For this review, take the finished solid that the model builds, in its own axes (mm). A direction names the side the tool comes from. Give positions to 0.01 mm unless a question says otherwise; leave off trailing zeros. Order: outer loops, then holes, each group sorted by start corner. A loop starts at its lowest first (then second) coordinate and runs counter-clockwise, first axis right, second up.
from build123d import *

# Parameters (mm, degrees)
F1_DEPTH = 25


with BuildPart() as f1:
    # F0 (on Front) → F1 (new body)
    with BuildSketch(Plane.XZ):
        with BuildLine():
            Line((27.1333980914, 4.2735439138), (-126.4131814241, 56.7106418312))
            Line((-126.4131814241, 56.7106418312), (-126.4131814241, 50.1115843654))
            Line((-126.4131814241, 50.1115843654), (-100.4294008017, -78.9824649692))
            Line((-100.4294008017, -78.9824649692), (109.0906560421, -23.7153619528))
            Line((109.0906560421, -23.7153619528), (31.3300916134, 2.8403473566))
            add(Edge.make_bspline(
                [(31.3300916134, 2.8403473566), (31.6087331931, 2.6379324169), (31.8639740687, 2.4078315454)],
                knots=[0.879679153, 0.879679153, 0.879679153, 1, 1, 1], degree=2))
            add(Edge.make_bspline(
                [(31.8639740687, 2.4078315454), (33.9853094976, 0.4954374993), (33.9853094976, -2.7315460807)],
                knots=[0, 0, 0, 1, 1, 1], degree=2))
            add(Edge.make_bspline(
                [(33.9853094976, -2.7315460807), (33.9853094976, -5.2562544572), (32.5691512359, -7.7229235606)],
                knots=[0, 0, 0, 1, 1, 1], degree=2))
            add(Edge.make_bspline(
                [(32.5691512359, -7.7229235606), (31.1529929742, -10.1895926641), (27.2759695363, -13.9621454105)],
                knots=[0, 0, 0, 1, 1, 1], degree=2))
            Line((27.2759695363, -13.9621454105), (21.4720422341, -19.6383863121))
            Line((21.4720422341, -19.6383863121), (21.4720422341, -19.7834844946))
            Line((21.4720422341, -19.7834844946), (35.1112713943, -19.7834844946))
            Line((35.1112713943, -19.7834844946), (35.1112713943, -22.575173527))
            Line((35.1112713943, -22.575173527), (17.6820777057, -22.575173527))
            Line((17.6820777057, -22.575173527), (17.6820777057, -19.9808180229))
            Line((17.6820777057, -19.9808180229), (24.6642022503, -12.9638699145))
            add(Edge.make_bspline(
                [(24.6642022503, -12.9638699145), (27.8563622665, -9.7310824072), (28.8720495444, -8.3526496729)],
                knots=[0, 0, 0, 1, 1, 1], degree=2))
            add(Edge.make_bspline(
                [(28.8720495444, -8.3526496729), (29.8877368223, -6.9742169386), (30.3955804612, -5.6683332956)],
                knots=[0, 0, 0, 1, 1, 1], degree=2))
            add(Edge.make_bspline(
                [(30.3955804612, -5.6683332956), (30.9034241002, -4.3624496526), (30.9034241002, -2.8592324814)],
                knots=[0, 0, 0, 1, 1, 1], degree=2))
            add(Edge.make_bspline(
                [(30.9034241002, -2.8592324814), (30.9034241002, -0.7349950888), (29.6149522391, 0.5070453539)],
                knots=[0, 0, 0, 1, 1, 1], degree=2))
            add(Edge.make_bspline(
                [(29.6149522391, 0.5070453539), (28.326480378, 1.7490857966), (26.0397330209, 1.7490857966)],
                knots=[0, 0, 0, 1, 1, 1], degree=2))
            add(Edge.make_bspline(
                [(26.0397330209, 1.7490857966), (24.3914176671, 1.7490857966), (22.911416205, 1.2035166302)],
                knots=[0, 0, 0, 1, 1, 1], degree=2))
            add(Edge.make_bspline(
                [(22.911416205, 1.2035166302), (21.4314147429, 0.6579474638), (19.6205894247, -0.7756225799)],
                knots=[0, 0, 0, 1, 1, 1], degree=2))
            Line((19.6205894247, -0.7756225799), (18.0245094165, 1.2731637578))
            add(Edge.make_bspline(
                [(18.0245094165, 1.2731637578), (21.6867875442, 4.3202255915), (26.0049094571, 4.3202255915)],
                knots=[0, 0, 0, 1, 1, 1], degree=2))
            add(Edge.make_bspline(
                [(26.0049094571, 4.3202255915), (26.5888819187, 4.3202255915), (27.1333980914, 4.2735439138)],
                knots=[0, 0, 0, 0.156237232, 0.156237232, 0.156237232], degree=2))
        make_face()
        Polygon((-78.7617822753, 1.2035166302), (-78.7617822753, -22.575173527), (-81.8436676727, -22.575173527), (-81.8436676727, 1.2035166302), (-90.241950479, 1.2035166302), (-90.241950479, 3.9429703168), (-70.3634994689, 3.9429703168), (-70.3634994689, 1.2035166302), align=None, mode=Mode.SUBTRACT)
        Polygon((-51.5877946463, -19.8183080584), (-51.5877946463, -22.575173527), (-66.370397485, -22.575173527), (-66.370397485, 3.9429703168), (-51.5877946463, 3.9429703168), (-51.5877946463, 1.2035166302), (-63.2885120875, 1.2035166302), (-63.2885120875, -7.3398643587), (-52.2958737771, -7.3398643587), (-52.2958737771, -10.0619062634), (-63.2885120875, -10.0619062634), (-63.2885120875, -19.8183080584), align=None, mode=Mode.SUBTRACT)
        with BuildLine():
            add(Edge.make_bspline(
                [(-28.3372618736, 0.1530057885), (-31.3495001434, 1.5633601229), (-34.3617384133, 1.5633601229)],
                knots=[0, 0, 0, 1, 1, 1], degree=2))
            add(Edge.make_bspline(
                [(-34.3617384133, 1.5633601229), (-38.7320956719, 1.5633601229), (-41.2626079756, -1.3473094191)],
                knots=[0, 0, 0, 1, 1, 1], degree=2))
            add(Edge.make_bspline(
                [(-41.2626079756, -1.3473094191), (-43.7931202794, -4.2579789612), (-43.7931202794, -9.3190035687)],
                knots=[0, 0, 0, 1, 1, 1], degree=2))
            add(Edge.make_bspline(
                [(-43.7931202794, -9.3190035687), (-43.7931202794, -14.5193224315), (-41.3525688488, -17.360344846)],
                knots=[0, 0, 0, 1, 1, 1], degree=2))
            add(Edge.make_bspline(
                [(-41.3525688488, -17.360344846), (-38.9120174182, -20.2013672604), (-34.3965619771, -20.2013672604)],
                knots=[0, 0, 0, 1, 1, 1], degree=2))
            add(Edge.make_bspline(
                [(-34.3965619771, -20.2013672604), (-31.6222847266, -20.2013672604), (-28.0644772904, -19.2030917644)],
                knots=[0, 0, 0, 1, 1, 1], degree=2))
            Line((-28.0644772904, -19.2030917644), (-28.0644772904, -21.9019179599))
            add(Edge.make_bspline(
                [(-28.0644772904, -21.9019179599), (-30.8213427589, -22.940820947), (-34.8666800886, -22.940820947)],
                knots=[0, 0, 0, 1, 1, 1], degree=2))
            add(Edge.make_bspline(
                [(-34.8666800886, -22.940820947), (-40.7228427365, -22.940820947), (-43.9062968618, -19.3830135108)],
                knots=[0, 0, 0, 1, 1, 1], degree=2))
            add(Edge.make_bspline(
                [(-43.9062968618, -19.3830135108), (-47.089750987, -15.8252060745), (-47.089750987, -9.2783760776)],
                knots=[0, 0, 0, 1, 1, 1], degree=2))
            add(Edge.make_bspline(
                [(-47.089750987, -9.2783760776), (-47.089750987, -5.1808034023), (-45.5575141793, -2.0989180048)],
                knots=[0, 0, 0, 1, 1, 1], degree=2))
            add(Edge.make_bspline(
                [(-45.5575141793, -2.0989180048), (-44.0252773715, 0.9829673927), (-41.1320196113, 2.6515964921)],
                knots=[0, 0, 0, 1, 1, 1], degree=2))
            add(Edge.make_bspline(
                [(-41.1320196113, 2.6515964921), (-38.2387618512, 4.3202255915), (-34.3211109222, 4.3202255915)],
                knots=[0, 0, 0, 1, 1, 1], degree=2))
            add(Edge.make_bspline(
                [(-34.3211109222, 4.3202255915), (-30.1538911192, 4.3202255915), (-27.0313782306, 2.7995966383)],
                knots=[0, 0, 0, 1, 1, 1], degree=2))
            Line((-27.0313782306, 2.7995966383), (-28.3372618736, 0.1530057885))
        make_face(mode=Mode.SUBTRACT)
        Polygon((-14.1176399831, 1.2035166302), (-14.1176399831, -22.575173527), (-17.1995253806, -22.575173527), (-17.1995253806, 1.2035166302), (-25.5978081869, 1.2035166302), (-25.5978081869, 3.9429703168), (-5.7193571768, 3.9429703168), (-5.7193571768, 1.2035166302), align=None, mode=Mode.SUBTRACT)
        with BuildLine():
            add(Edge.make_bspline(
                [(10.734776725, 2.552929728), (12.8764258995, 0.7856338644), (12.8764258995, -2.2962515331)],
                knots=[0, 0, 0, 1, 1, 1], degree=2))
            add(Edge.make_bspline(
                [(12.8764258995, -2.2962515331), (12.8764258995, -4.8383716914), (11.4515617468, -6.4518634814)],
                knots=[0, 0, 0, 1, 1, 1], degree=2))
            add(Edge.make_bspline(
                [(11.4515617468, -6.4518634814), (10.0266975941, -8.0653552715), (7.4149303081, -8.6109244379)],
                knots=[0, 0, 0, 1, 1, 1], degree=2))
            Line((7.4149303081, -8.6109244379), (7.4149303081, -8.7560226204))
            add(Edge.make_bspline(
                [(7.4149303081, -8.7560226204), (10.6070903243, -9.150689677), (12.148033023, -10.7844952125)],
                knots=[0, 0, 0, 1, 1, 1], degree=2))
            add(Edge.make_bspline(
                [(12.148033023, -10.7844952125), (13.6889757218, -12.4183007481), (13.6889757218, -15.0648915979)],
                knots=[0, 0, 0, 1, 1, 1], degree=2))
            add(Edge.make_bspline(
                [(13.6889757218, -15.0648915979), (13.6889757218, -18.8548561263), (11.0597966539, -20.8978385367)],
                knots=[0, 0, 0, 1, 1, 1], degree=2))
            add(Edge.make_bspline(
                [(11.0597966539, -20.8978385367), (8.430617586, -22.940820947), (3.5901422159, -22.940820947)],
                knots=[0, 0, 0, 1, 1, 1], degree=2))
            add(Edge.make_bspline(
                [(3.5901422159, -22.940820947), (1.4833166052, -22.940820947), (-0.2665674764, -22.6216049454)],
                knots=[0, 0, 0, 1, 1, 1], degree=2))
            add(Edge.make_bspline(
                [(-0.2665674764, -22.6216049454), (-2.016451558, -22.3023889438), (-3.6647669118, -21.5072509034)],
                knots=[0, 0, 0, 1, 1, 1], degree=2))
            Line((-3.6647669118, -21.5072509034), (-3.6647669118, -18.6401108161))
            add(Edge.make_bspline(
                [(-3.6647669118, -18.6401108161), (-1.9410005031, -19.4932881295), (0.0091190705, -19.9372885681)],
                knots=[0, 0, 0, 1, 1, 1], degree=2))
            add(Edge.make_bspline(
                [(0.0091190705, -19.9372885681), (1.959238644, -20.3812890068), (3.7004168347, -20.3812890068)],
                knots=[0, 0, 0, 1, 1, 1], degree=2))
            add(Edge.make_bspline(
                [(3.7004168347, -20.3812890068), (10.5722667605, -20.3812890068), (10.5722667605, -14.9952444703)],
                knots=[0, 0, 0, 1, 1, 1], degree=2))
            add(Edge.make_bspline(
                [(10.5722667605, -14.9952444703), (10.5722667605, -10.1663769549), (2.9923377038, -10.1663769549)],
                knots=[0, 0, 0, 1, 1, 1], degree=2))
            Line((2.9923377038, -10.1663769549), (0.3805704178, -10.1663769549))
            Line((0.3805704178, -10.1663769549), (0.3805704178, -7.5778253781))
            Line((0.3805704178, -7.5778253781), (3.0271612676, -7.5778253781))
            add(Edge.make_bspline(
                [(3.0271612676, -7.5778253781), (6.126458447, -7.5778253781), (7.9401857289, -6.2080985347)],
                knots=[0, 0, 0, 1, 1, 1], degree=2))
            add(Edge.make_bspline(
                [(7.9401857289, -6.2080985347), (9.7539130109, -4.8383716914), (9.7539130109, -2.4065261518)],
                knots=[0, 0, 0, 1, 1, 1], degree=2))
            add(Edge.make_bspline(
                [(9.7539130109, -2.4065261518), (9.7539130109, -0.4680144329), (8.421911695, 0.6405356819)],
                knots=[0, 0, 0, 1, 1, 1], degree=2))
            add(Edge.make_bspline(
                [(8.421911695, 0.6405356819), (7.0899103792, 1.7490857966), (4.8031630221, 1.7490857966)],
                knots=[0, 0, 0, 1, 1, 1], degree=2))
            add(Edge.make_bspline(
                [(4.8031630221, 1.7490857966), (3.0619848314, 1.7490857966), (1.5210421327, 1.2760657215)],
                knots=[0, 0, 0, 1, 1, 1], degree=2))
            add(Edge.make_bspline(
                [(1.5210421327, 1.2760657215), (-0.0199005661, 0.8030456463), (-1.9990397761, -0.4680144329)],
                knots=[0, 0, 0, 1, 1, 1], degree=2))
            Line((-1.9990397761, -0.4680144329), (-3.5196687293, 1.5633601229))
            add(Edge.make_bspline(
                [(-3.5196687293, 1.5633601229), (-1.8887651574, 2.851831984), (0.2412761625, 3.5860287877)],
                knots=[0, 0, 0, 1, 1, 1], degree=2))
            add(Edge.make_bspline(
                [(0.2412761625, 3.5860287877), (2.3713174825, 4.3202255915), (4.7335158945, 4.3202255915)],
                knots=[0, 0, 0, 1, 1, 1], degree=2))
            add(Edge.make_bspline(
                [(4.7335158945, 4.3202255915), (8.5931275504, 4.3202255915), (10.734776725, 2.552929728)],
                knots=[0, 0, 0, 1, 1, 1], degree=2))
        make_face(mode=Mode.SUBTRACT)
    extrude(amount=F1_DEPTH)


solid = f1.part
1) Clearance check with flat-ended pins moving along their axes: pin 1 (3 mm diameter, centred on x = -56.5, y = -16.5, fed in from +Z); pin 2 (0.8 mm diameter, centred on y = -14.5, z = -21, fed in from -X); pin 3 (12 mm diameter, centred on x = -54, y = -14.5, fed in from +Z). State where each tip first meets the part, or that it passes through.
Answer sheet:
pin 1: stops at z = 33.35
pin 2: stops at x = -112.18
pin 3: stops at z = 34.03
2) Draft analysis for pull direction X (two halves, no side actions). For faces 3 (the face through (-126.413, -12, 53)), 4 (the face through (70.75, -12.32, -10.62)), 5 (the face through (-36, 0, -10)), 6 (the face through (27, -12, -22.575)), state which applies: +X half, -X half, draft (parallel to the pull), parting line (faces both ways), or undercut.
Answer sheet:
face 3: -X half
face 4: +X half
face 5: draft
face 6: undercut
3) We need section C-C on x = 66. Give the boundary of the cut face in (y, z).
Answer sheet:
outline: (-25, -35.08) - (0, -35.08) - (0, -9) - (-25, -9) - close
4) To check wall thickness, follow line 1 (Z direction, x = 8, y = -11); line 2 (Z direction, x = 29.5, y = -20); line 3 (Z direction, x = 21, y = -22.25). State the ranges of each line that lie inside material, in increasing order.
Answer sheet:
line 1: z = -50.38 to -22.4, -19.57 to -11.01, -8.84 to -8.47, -6.16 to 0.95, 3.92 to 10.81
line 2: z = -44.71 to -22.58, -19.78 to -11.69, -7.43 to 0.61
line 3: z = -46.95 to -22.58, -16.65 to 0.22, 3.2 to 6.37
5) Tool access review of faces 1 (the face through (2.864, -12.325, -51.736)), 2 (the face through (-58, -12, -10.062)): name each direction out of +Z, -Z, +X, -X, +Y, -Y from which nothing blocks a thin tool from reaching the whole face with its end or side.
Answer sheet:
face 1: -Z, +X, +Y, -Y
face 2: +Y, -Y
6) We need section B-B on z = 23.5. Give the boundary of the cut face in (x, y).
Answer sheet:
outline: (-121.06, -25) - (-29.17, -25) - (-29.17, 0) - (-121.06, 0) - close
7) We need section A-A on y = -21. Count the separate pieces of the cut face and the enclosed holes in it, then the cut area to 3 significant figures.
Answer sheet:
separate pieces: 1
enclosed holes: 5
area: 14,100 mm2
